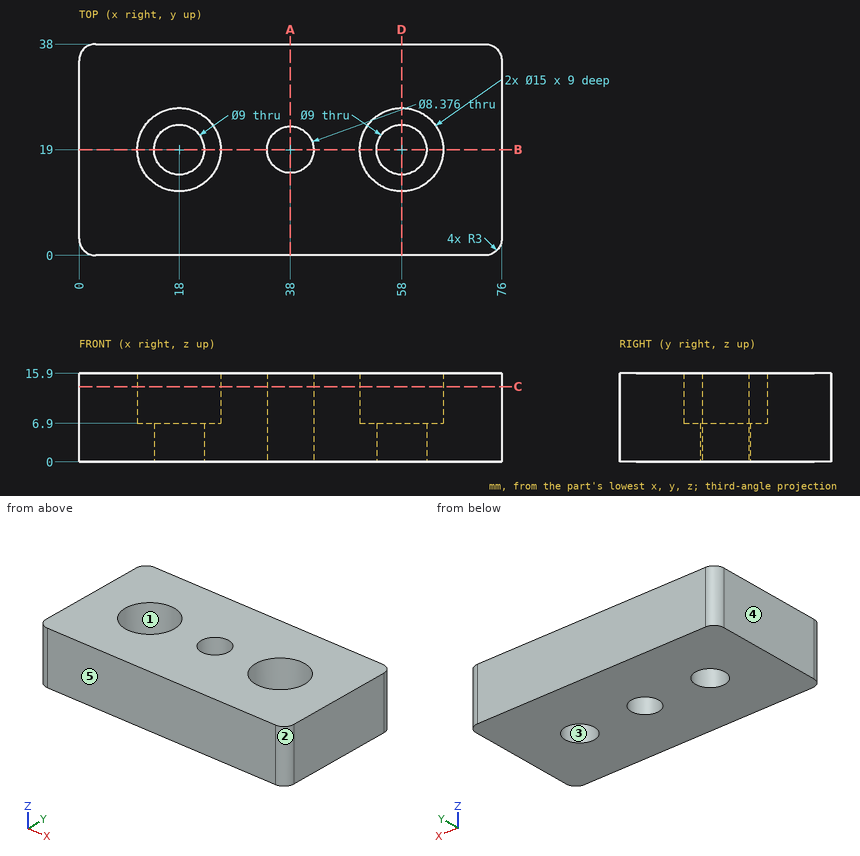
Job drawing, mm, ordinate dimensions from the low corner. One solid piece. A direction names the side the tool comes from. Coordinates: 2 decimals unless noted, no trailing zeros. Loops run counter-clockwise (first coordinate to the right, second up) from the corner with the lowest first, then second, coordinate; pieces in that order, holes last. Notation, with made-up numbers: (-17, 33) -> (0, 33) arc R19 ccw to (0, 64) -> close; hole circle Ø7 at (-36.75, 23). An arc over 180 degrees is marked (long way). One line per item, written item: value.
1. Drill centre lines: line 1 (X direction, y = 19, z = 11.25); line 2 (X direction, y = 19, z = 4); line 3 (Y direction, x = 58, z = 4). Where is each one in solid material? Low to high. Write a range as [from, to].
Answers:
line 1: x = [0, 10.5], [25.5, 33.81], [42.19, 50.5], [65.5, 76]
line 2: x = [0, 13.5], [22.5, 33.81], [42.19, 53.5], [62.5, 76]
line 3: y = [0, 14.5], [23.5, 38]
2. Which spindle directions (+Z, -Z, +X, -X, +Y, -Y) get a long thin tool onto all of the face, cutting with end or side? Do the marked faces 1 and 2. Say none if no direction does.
Answers:
face 1: +Z
face 2: +Z, -Z, +X, -Y
3. Slice it at C-C on z = 13.5. Write the cut outline in (x, y), and give its area (3 significant figures).
Answers:
outline: (0, 3) arc R3 ccw to (3, 0) -> (73, 0) arc R3 ccw to (76, 3) -> (76, 35) arc R3 ccw to (73, 38) -> (3, 38) arc R3 ccw to (0, 35) -> close; hole circle Ø15 at (18, 19); hole circle Ø8.38 at (38, 19); hole circle Ø15 at (58, 19)
area: 2,470 mm^2
4. Slice it at B-B on y = 19. Write the cut outline in (x, z), and give its area (3 significant figures).
Answers:
outline: (0, 0) -> (13.5, 0) -> (13.5, 6.9) -> (10.5, 6.9) -> (10.5, 15.9) -> (0, 15.9) -> close; (22.5, 0) -> (33.81, 0) -> (33.81, 15.9) -> (25.5, 15.9) -> (25.5, 6.9) -> (22.5, 6.9) -> close; (42.19, 0) -> (53.5, 0) -> (53.5, 6.9) -> (50.5, 6.9) -> (50.5, 15.9) -> (42.19, 15.9) -> close; (62.5, 0) -> (76, 0) -> (76, 15.9) -> (65.5, 15.9) -> (65.5, 6.9) -> (62.5, 6.9) -> close
area: 681 mm^2
5. Flat gauge pins, fed straight in: P1, Ø1, axis at x = 21.5, y = 13.5, coming from the +Z side; P2, Ø7, axis at x = 58, y = 19, coming from the -Z side. Where does each tip first touch, or does it go through?
Answers:
P1: stops at z = 6.9
P2: passes through
6. Slice it at A-A on x = 38. Write the cut outline in (y, z).
Answers:
outline: (0, 0) -> (14.81, 0) -> (14.81, 15.9) -> (0, 15.9) -> close; (23.19, 0) -> (38, 0) -> (38, 15.9) -> (23.19, 15.9) -> close
7. Pull direction X, two halves, no side cores. Call the marked faces 3, 4 and 5: pulls with the +X half, pulls with the -X half, needs draft (parallel to the pull), parting line crosses it, or undercut.
Answers:
face 3: undercut
face 4: pulls with the -X half
face 5: needs draft
8. Slice it at D-D on x = 58. Write the cut outline in (y, z).
Answers:
outline: (0, 0) -> (14.5, 0) -> (14.5, 6.9) -> (11.5, 6.9) -> (11.5, 15.9) -> (0, 15.9) -> close; (23.5, 0) -> (38, 0) -> (38, 15.9) -> (26.5, 15.9) -> (26.5, 6.9) -> (23.5, 6.9) -> close
